Design review of the part built by this model. Coordinates are the model's own, in mm. Face numbers are marked on the shaded views. A direction names the side the tool comes from. Give positions to 0.01 mm unless a question says otherwise; leave off trailing zeros. Order: outer loops, then holes, each group sorted by start corner. A loop starts at its lowest first (then second) coordinate and runs counter-clockwise, first axis right, second up. Notation, with made-up numbers: (-2.5, 0.5) -> (29.5, 0.5) arc R23 ccw to (29.5, 31.5) -> close; hole circle Ø3 at (48.25, 58.25). An arc over 180 degrees is marked (long way). One line per item, written item: value.
from build123d import *

# Parameters (mm, degrees)
F0_W     = 50
F0_H     = 50
F1_DEPTH = 1
F2_W     = 2.719909
F2_H     = 45.7574
F3_DEPTH = 10
F4_W     = 2.818288
F4_H     = 33.003134
F5_DEPTH = 10
F6_W     = 17.629229
F6_H     = 3.787741
F7_DEPTH = 10
F9_DEPTH = 10


with BuildPart() as f1:
    # F0 (on Top) → F1 (new body)
    with BuildSketch(Plane.XY):
        Rectangle(F0_W, F0_H)
    extrude(amount=F1_DEPTH)

    # F2 (on face) → F3 (join)
    with BuildSketch(Plane.XY.offset(1)):
        with Locations((22.101672, -0.088033)):
            Rectangle(F2_W, F2_H)
    extrude(amount=F3_DEPTH)

    # F4 (on face) → F5 (join)
    with BuildSketch(Plane.XY.offset(1)):
        with Locations((-22.33317, -6.452603)):
            Rectangle(F4_W, F4_H)
    extrude(amount=F5_DEPTH)

    # F6 (on face) → F7 (join)
    with BuildSketch(Plane.XY.offset(1)):
        with Locations((-4.384833, -20.898708)):
            Rectangle(F6_W, F6_H)
    extrude(amount=F7_DEPTH)

    # F8 (on face) → F9 (join)
    with BuildSketch(Plane(origin=(0, 25, 0), x_dir=(-1, 0, 0), z_dir=(0, 1, 0))):
        with BuildLine():
            Line((2.223496, 1), (14.291007, 1))
            ThreePointArc((14.291007, 1), (8.257251, 7.033755), (2.223496, 1))
        make_face()
    extrude(amount=-F9_DEPTH)


solid = f1.part
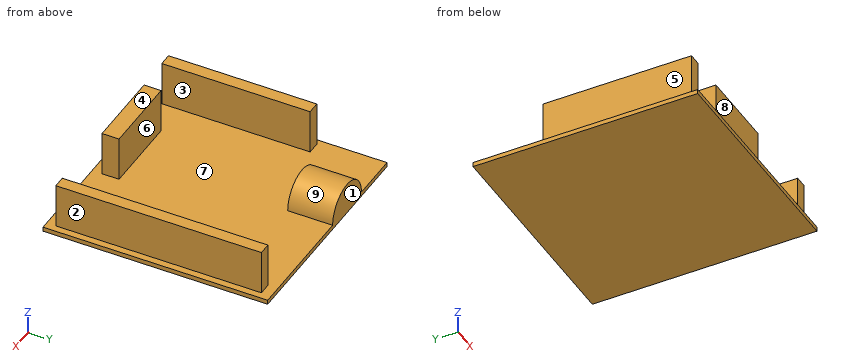
Item 1: Add section C-C on x = -7.5. Give the boundary of the cut face in (y, z).
Returned:
outline: (-25, 0) -> (25, 0) -> (25, 6.99) -> (15, 6.99) -> (15, 1) -> (-19, 1) -> (-19, 11) -> (-22.79, 11) -> (-22.79, 1) -> (-25, 1) -> close
Item 2: Add section A-A on z = 6. Give the boundary of the cut face in (x, y).
Returned:
outline: (-23.74, -22.95) -> (-20.92, -22.95) -> (-20.92, 10.05) -> (-23.74, 10.05) -> close; (-13.2, -22.79) -> (4.43, -22.79) -> (4.43, -19) -> (-13.2, -19) -> close; (-11.63, 15) -> (-4.88, 15) -> (-4.88, 25) -> (-11.63, 25) -> close; (20.74, -22.97) -> (23.46, -22.97) -> (23.46, 22.79) -> (20.74, 22.79) -> close
Item 3: To check wall thickness, follow line 1 along X through (y, z) = (-17, 5); line 2 along Y through (x, z) = (-7, 4.5); line 3 along Y through (x, z) = (3.5, 8.75). State the ranges of each line that lie inside material, in increasing order. Write a range as from..to.
Returned:
line 1: -23.74..-20.92, 20.74..23.46
line 2: -22.79..-19, 15..25
line 3: -22.79..-19
Item 4: Draft analysis for pull direction Y (two halves, no side actions). For the marked faces 6, 7, 8 and 9, state which applies: pulls with the +Y half, pulls with the -Y half, needs draft (parallel to the pull), parting line crosses it, or undercut.
Returned:
face 6: undercut
face 7: undercut
face 8: pulls with the -Y half
face 9: needs draft
Item 5: Add section D-D on y = -6. Give the boundary of the cut face in (x, z), plus the area to 3 significant figures.
Returned:
outline: (-25, 0) -> (25, 0) -> (25, 1) -> (23.46, 1) -> (23.46, 11) -> (20.74, 11) -> (20.74, 1) -> (-20.92, 1) -> (-20.92, 11) -> (-23.74, 11) -> (-23.74, 1) -> (-25, 1) -> close
area: 105 mm²
Item 6: Clearance check with flat-ended pins moving along their axes: P1, Ø5, axis at x = 13, y = 17.5, coming from the +Z side; P2, Ø5, axis at y = -9, z = 4.5, coming from the -X side; P3, Ø6, axis at x = -0.5, y = 5, coming from the -Z side; P4, Ø2.5, axis at x = -22, z = 7, coming from the -Y side. State where each tip first meets the part, or that it passes through.
Returned:
P1: z = 1
P2: x = -23.74
P3: z = 0
P4: y = -22.95
Item 7: Add section B-B on y = 18.5. Give the boundary of the cut face in (x, z), plus the area to 3 significant figures.
Returned:
outline: (-25, 0) -> (25, 0) -> (25, 1) -> (23.46, 1) -> (23.46, 11) -> (20.74, 11) -> (20.74, 1) -> (-2.22, 1) arc R6.03 ccw to (-14.29, 1) -> (-25, 1) -> close
area: 134 mm²
Item 8: Machinability: for the marked faces 1, 2, 3, 4 and 5, which of the approach directions +Z, -Z, +X, -X, +Y, -Y give a long, thin tool a straight path to every point of the face, cutting with its end or side? Answer none if there is none.
Returned:
face 1: +Z, -Z, +X, -X, +Y
face 2: +Z, +X, +Y, -Y
face 3: +Z, +Y, -Y
face 4: +Z, +X, -X, +Y, -Y
face 5: +Z, -X, +Y, -Y
